Autodesk Inventor part; units mm, degrees
ref_plane "Work Plane1" through (60, 0, 0) normal (0, 0, 1) x (1, 0, 0)
ref_plane "YZ Plane" through (0, 0, 0) normal (1, 0, 0) x (0, 1, 0)
ref_plane "XZ Plane" through (0, 0, 0) normal (0, 1, 0) x (-1, 0, 0)
sketch "Boceto1" plane through (0, 0, 0) normal (0, 0, 1) x (1, 0, 0)
  line L0 (0, 1.7526) -> (31.75, 1.7526)
  line L1 (31.75, 1.7526) -> (31.75, 0)
  line L2 (31.75, 0) -> (0, 0)
  line L3 (-6.35, 0) -> (38.1, 0)
  line L4 (0, -0.3505) -> (0, 2.1031)
  line L5 (0, 1.7526) -> (0, 0)
  dimension "d1" = 3.5052
  dimension "d52" = 31.75
revolve "Cuerpo" add sketch "Boceto1" angle 360 about axis through (31.75, 0, 0) along (-1, 0, 0)
sketch "Boceto2" plane through (0, 0, 0) normal (-1, 0, 0) x (0, 0, 1)
  line L0 (0, 3.6662) -> (3.175, 1.8331)
  line L1 (3.175, 1.8331) -> (3.175, -1.8331)
  line L2 (3.175, -1.8331) -> (0, -3.6662)
  line L3 (0, -3.6662) -> (-3.175, -1.8331)
  line L4 (-3.175, -1.8331) -> (-3.175, 1.8331)
  line L5 (-3.175, 1.8331) -> (0, 3.6662)
  line L6 (-4.445, 0) -> (4.445, 0)
  line L7 (0, 5.1326) -> (0, -5.1326)
  point P0 (0, 0)
  point P1 (0, 0)
  dimension "d10" = 6.35
extrude "Cabeza" add sketch "Boceto2" along normal blind 2.3622
sketch "Boceto3" plane through (0, 0, 0) normal (0, 0, 1) x (1, 0, 0)
  line L0 (-2.3622, 0.6096) -> (-1.1938, 0.6096)
  line L1 (-1.1938, 0.6096) -> (-1.1938, -0.6096)
  line L2 (-1.1938, -0.6096) -> (-2.3622, -0.6096)
  line L3 (-2.3622, -0.6096) -> (-2.3622, 0.6096)
  line L4 (-1.1938, 0) -> (-2.3622, 0) construction
  line L5 (-2.5959, 0) -> (-0.9601, 0)
  line L6 (-2.3622, 1.8331) -> (-2.3622, -1.8331)
  dimension "d11" = 1.2192
  dimension "d13" = 1.1684
extrude "Ranura" cut sketch "Boceto3" along normal through all both and the other way through all
sketch "Boceto4" plane through (0, 0, 0) normal (0, 0, 1) x (1, 0, 0)
  line L0 (-2.3622, 3.175) -> (-2.3622, 3.6662)
  line L1 (-2.3622, 3.6662) -> (-2.0786, 3.6662)
  line L2 (-2.0786, 3.6662) -> (-2.3622, 3.175)
  line L3 (-2.0786, 3.6662) -> (-2.3622, 3.6662)
  line L4 (-2.3622, 3.6662) -> (-2.3622, 3.175)
  line L5 (-2.3622, 3.6662) -> (-2.3622, 1.8331)
  line L6 (-2.8346, 0) -> (0.4724, 0)
  line L7 (0, 3.6662) -> (-2.3622, 3.6662)
  dimension "d4" = 30
  dimension "d17" = 6.35
revolve "Chaflán1" cut sketch "Boceto4" angle 360 about axis through (-10, 0, 0) along (1, 0, 0)
thread "Rosca"
chamfer "Chaflán2" distance 0.3975 distance2 0.3976 1 edges at (31.75, -1.7526, 0) measured on face at (31.75, 0.2072, -0.5462)
ref_plane "Work Plane1" through (60, 0, 0) normal (0, 0, 1) x (1, 0, 0)
equation "\"d1\" = GD"
equation "\"d52\" = NLG"
equation "\"d10\" = SW"
equation "\"d2\" = KOH - SD"
equation "\"d11\" = SBR"
equation "\"d13\" = STI"
equation "\"d4\" = ANG1"
equation "\"d17\" = SW0"
equation "\"d15\" = GEL"
equation "\"d5\" = -0.5 * SPD + 0.5 * GD"
equation "\"NLG\" = 31.75"
equation "\"GD\" = NND"
equation "\"KOH\" = 2.3622"
equation "\"GEL\" = 31.26232"
equation "\"SW\" = 6.35"
equation "\"SW0\" = 6.35"
equation "\"SPD\" = GD1"
equation "\"SD2\" = NND"
equation "\"SD\" = 0"
equation "\"ANG1\" = 30deg"
equation "\"GUL\" = -0.5 * GD1 + 0.5 * NND"
equation "\"STI\" = 1.1684"
equation "\"SBR\" = 1.2192"
equation "\"RR\" = 0.39751"
equation "\"THREADDIA\" = 3.5052"
equation "\"TOA\" = 30deg"
equation "\"BDM\" = NND"
equation "\"FAWI\" = 45deg"
equation "\"NND\" = 3.5052"
equation "\"E0\" = 1.155 * SW"
equation "\"GAL\" = 0.39751"
equation "\"GD1\" = 2.71018"
properties part number "ANSI B18.6.3 - Nº 6 - 32 x 1 1/4" material "Acero, suave"
Read the model definition and answer for the solid it produces. Units are mm, in the model's axes. A direction names the side the tool comes from. Round coordinates to 2 decimals unless told otherwise and drop trailing zeros. Write each loop counter-clockwise with the first axis right and the second up, starting at its lowest first coordinate (ties: lowest second). Pieces come first, ordered by that corner, then holes.
1. Straight lines are drawn through the part: L1, parallel to X at y = -1.5, z = -1.75; L2, parallel to Z at x = 23, y = 0; L3, parallel to X at y = 0.25, z = 1. For each, find the intervals that lie inside material, in ascending order.
2. The part is cut by section A-A, the plane y = 0. Determine the outline of the cut face in (x, z) (3 decimals).
3. Which of the six approach directions +Z, -Z, +X, -X, +Y, -Y give full straight-line access (tool end or side, diameter ignored) to faces 1 (the face through (-2, 0.61, 0)), 2 (the face through (-2.362, -2, 0)), 3 (the face through (0, 2, 1))?
4. Determine the mould class of faces 4 (the face through (-1.194, 0, 0)), 5 (the face through (31.75, 0, 0)), 6 (the face through (-1.16, -2.76, -1.57)), 7 (the face through (-2, -0.61, 0)) for opening direction Y: pulls with the +Y half, pulls with the -Y half, needs draft (parallel to the pull), parting line crosses it, or undercut.
5. Given pin 1 Ø3 at (x, y) = (17.5, -2.5) entering from +Z; pin 2 Ø1.5 at (x, y) = (9, -2) entering from -Z; pin 3 Ø1.3 at (x, z) = (-2, -1) entering from -Y, each flat-ended and moving along its own axis, determine where each tip first touches the part or whether it passes through.
6. The part is cut by section B-B, the plane x = 15. Determine the outline of the cut face in (y, z), then the cut area to 3 significant figures.
Values:
1. L1: x = -2.36 to 0
1. L2: z = -1.75 to 1.75
1. L3: x = -1.19 to 31.75
2. outline: (-1.194, -3.175) - (0, -3.175) - (0, -1.753) - (31.352, -1.753) - (31.75, -1.355) - (31.75, 1.355) - (31.352, 1.753) - (0, 1.753) - (0, 3.175) - (-1.194, 3.175) - close
3. face 1: +Z, -Z, -X
3. face 2: +Z, -Z, -X, +Y, -Y
3. face 3: +X
4. face 4: undercut
4. face 5: needs draft
4. face 6: pulls with the -Y half
4. face 7: undercut
5. pin 1: stops at z = 1.44
5. pin 2: stops at z = -1.23
5. pin 3: stops at y = -3.46
6. outline: circle Ø3.51 at (0, 0)
6. area: 9.65 mm2
